Part model, mm, in its own coordinate system. A direction names the side the tool comes from. Give positions to 0.01 mm unless a question says otherwise; leave off trailing zeros. Order: outer loops, then holes, each group sorted by start corner. A loop starts at its lowest first (then second) coordinate and runs counter-clockwise, first axis right, second up.
1. Slice it at D-D on y = 29. List the corners of the cut face in (x, z).
2. Slice it at B-B on y = 0. List the corners of the cut face in (x, z).
3. Slice it at C-C on x = -34.43. List the corners of the cut face in (y, z).
4. Slice it at A-A on x = -0.5. List the corners of the cut face in (y, z), and give its area (3 significant figures).
5. Drop flat-ended pins along their axis: pin 1 Ø5 at (y, z) = (38, 3.5) entering from +X; pin 2 Ø2.5 at (x, z) = (-5, 3) entering from +Y; pin 3 Ø4 at (y, z) = (38.5, 5) entering from -X. Give the stop position or say it passes through.
6. Mould opens along X. For faces 6 (the flat face through (22, 52, 4)), 7 (the flat face through (0, 41, 4)), 8 (the flat face through (7, -7, 2)), 9 (the flat face through (-22, 52, 4)) say: +X half, -X half, draft (parallel to the pull), parting line (faces both ways), or undercut.
7. Which spindle directions (+Z, -Z, +X, -X, +Y, -Y) get a long thin tool onto all of the face, cutting with end or side? Do faces 1 (the cylindrical face through (9.824, 3.094, 1.458)), 2 (the flat face through (-1, 14, 0)), 3 (the cylindrical face through (4.38, -8.43, 0.46)), 4 (the flat face through (-15, 14, 6)), 5 (the flat face through (13, 46, 4)). Say none if no direction does.
8. Probe line 1 (Y direction, x = -45.5, z = 7.75); line 2 (Y direction, x = 15, z = 2); line 3 (Y direction, x = 16, z = 3.15). List the from-to ranges inside material, lowest first.
from build123d import *

# Parameters (mm, degrees)
SKETCH_2_W                = 100
SKETCH_2_H                = 40
EXTRUDE_1_DEPTH           = 6
SKETCH_5_W                = 100
SKETCH_5_H                = 40
EXTRUDE_2_DEPTH           = 3
SKETCH_6_R                = 9.5
CUT_EXTRUDE_1_DEPTH       = 7
CUT_EXTRUDE_START         = -8
SKETCH_7_R                = 9.5
CUT_EXTRUDE_2_DEPTH       = 8
SKETCH_8_R                = 10.3
CUT_EXTRUDE_3_DEPTH       = 1.1
SKETCH_9_R                = 1.5
CUT_EXTRUDE_4_DEPTH       = 15
SKETCH_11_W               = 100
SKETCH_11_H               = 9
EXTRUDE_5_DEPTH           = 8
FILLET_3_R                = 5
SKETCH_16_R               = 1.5
CUT_EXTRUDE_6_DEPTH       = 10
HOLE_WIZARD_5_D           = 3
HOLE_WIZARD_5_CBORE_D     = 5.5
HOLE_WIZARD_5_CBORE_DEPTH = 3
SKETCH_20_R               = 1.5
CUT_EXTRUDE_7_DEPTH       = 10
SKETCH_22_R               = 9.5
SKETCH_22_R_2             = 8.5
EXTRUDE_6_DEPTH           = 2
SKETCH_23_W               = 46
SKETCH_23_H               = 8
EXTRUDE_7_DEPTH           = 25
SKETCH_24_W               = 13
SKETCH_24_H               = 8
CUT_EXTRUDE_8_DEPTH       = 12
CHAMFER_1_SIZE            = 2
FILLET_4_R                = 4
SKETCH_25_R               = 1.5
CUT_EXTRUDE_9_DEPTH       = 91.65870063


with BuildPart() as part:
    # 草图2 → 凸台-拉伸1 (new body)
    with BuildSketch(Plane.XY):
        Rectangle(SKETCH_2_W, SKETCH_2_H)
    extrude(amount=EXTRUDE_1_DEPTH)

    # 草图5 → 凸台-拉伸2 (add)
    with BuildSketch(Plane.XY.offset(6)):
        Rectangle(SKETCH_5_W, SKETCH_5_H)
    extrude(amount=EXTRUDE_2_DEPTH)

    # 草图6 → 切除-拉伸1 (cut)
    with BuildSketch(Plane.XY.offset(9)):
        Circle(SKETCH_6_R)
    extrude(amount=-CUT_EXTRUDE_1_DEPTH, mode=Mode.SUBTRACT)

    # 草图7 → 切除-拉伸2 (cut)
    with BuildSketch(Plane(origin=(0, 0, 0), x_dir=(-1, 0, 0), z_dir=(0, 0, -1)).offset(CUT_EXTRUDE_START)):
        with Locations(Location((0, 0, 0), (0, 0, 180))):
            Circle(SKETCH_7_R)
    extrude(amount=CUT_EXTRUDE_2_DEPTH, mode=Mode.SUBTRACT)

    # 草图8 → 切除-拉伸3 (cut)
    with BuildSketch(Plane.XY.offset(2)):
        Circle(SKETCH_8_R)
    extrude(amount=-CUT_EXTRUDE_3_DEPTH, mode=Mode.SUBTRACT)

    # 草图9 → 切除-拉伸4 (cut)
    with BuildSketch(Plane(origin=(0, 0, 0), x_dir=(-1, 0, 0), z_dir=(0, 0, -1))):
        with Locations((-15.07, 5)):
            Circle(SKETCH_9_R)
        with Locations((34.43, 5)):
            Circle(SKETCH_9_R)
        with Locations((-15.07, -5)):
            Circle(SKETCH_9_R)
        with Locations((34.43, -5)):
            Circle(SKETCH_9_R)
    extrude(amount=-CUT_EXTRUDE_4_DEPTH, mode=Mode.SUBTRACT)

    # 草图11 → 凸台-拉伸5 (add)
    with BuildSketch(Plane(origin=(0, 20, 0), x_dir=(1, 0, 0), z_dir=(0, 1, 0))):
        with Locations((0, -4.5)):
            Rectangle(SKETCH_11_W, SKETCH_11_H)
    extrude(amount=EXTRUDE_5_DEPTH)

    # 圆角3
    fillet_3_edges = [part.edges().sort_by_distance(p)[0] for p in [
        (-50, 28, 4.5),
        (50, 28, 4.5),
        (50, -20, 4.5),
        (-50, -20, 4.5),
    ]]
    fillet(fillet_3_edges, radius=FILLET_3_R)

    # 草图16 → 切除-拉伸6 (cut)
    with BuildSketch(Plane(origin=(0, 0, 0), x_dir=(-1, 0, 0), z_dir=(0, 0, -1))):
        with Locations((-6, 15.6)):
            Circle(SKETCH_16_R)
        with Locations((6, 15.6)):
            Circle(SKETCH_16_R)
        with Locations((-16, 15.6)):
            Circle(SKETCH_16_R)
        with Locations((16, 15.6)):
            Circle(SKETCH_16_R)
    extrude(amount=-CUT_EXTRUDE_6_DEPTH, mode=Mode.SUBTRACT)

    # 孔5 (through all)
    with Locations(Plane(origin=(-16, 15.6, 9), x_dir=(1, 0, 0), z_dir=(0, 0, 1))):
        with Locations((0, 0), (10, 0), (22, 0), (32, 0)):
            CounterBoreHole(HOLE_WIZARD_5_D / 2, HOLE_WIZARD_5_CBORE_D / 2, HOLE_WIZARD_5_CBORE_DEPTH)

    # 草图20 → 切除-拉伸7 (cut)
    with BuildSketch(Plane(origin=(0, 0, 0), x_dir=(-1, 0, 0), z_dir=(0, 0, -1))):
        with Locations((-46, 24)):
            Circle(SKETCH_20_R)
        with Locations((46, 24)):
            Circle(SKETCH_20_R)
        with Locations((-46, -16)):
            Circle(SKETCH_20_R)
        with Locations((46, -16)):
            Circle(SKETCH_20_R)
    extrude(amount=-CUT_EXTRUDE_7_DEPTH, mode=Mode.SUBTRACT)

    # 草图22 → 凸台-拉伸6 (add)
    with BuildSketch(Plane.XY.offset(9)):
        Circle(SKETCH_22_R)
        Circle(SKETCH_22_R_2, mode=Mode.SUBTRACT)
    extrude(amount=-EXTRUDE_6_DEPTH)

    # 草图23 → 凸台-拉伸7 (add)
    with BuildSketch(Plane(origin=(0, 28, 0), x_dir=(1, 0, 0), z_dir=(0, 1, 0))):
        with Locations((0, -4)):
            Rectangle(SKETCH_23_W, SKETCH_23_H)
    extrude(amount=EXTRUDE_7_DEPTH)

    # 草图24 → 切除-拉伸8 (cut)
    with BuildSketch(Plane(origin=(0, 53, 0), x_dir=(1, 0, 0), z_dir=(0, 1, 0))):
        with Locations((-6.5, -4)):
            Rectangle(SKETCH_24_W, SKETCH_24_H)
        with Locations((6.5, -4)):
            Rectangle(SKETCH_24_W, SKETCH_24_H)
    extrude(amount=-CUT_EXTRUDE_8_DEPTH, mode=Mode.SUBTRACT)

    # 倒角1
    chamfer_1_edges = [part.edges().sort_by_distance(p)[0] for p in [
        (-23, 53, 4),
        (23, 53, 4),
    ]]
    chamfer(chamfer_1_edges, length=CHAMFER_1_SIZE)

    # 圆角4
    fillet_4_edges = [part.edges().sort_by_distance(p)[0] for p in [
        (17, 53, 8),
        (17, 53, 0),
        (-17, 53, 8),
        (-17, 53, 0),
    ]]
    fillet(fillet_4_edges, radius=FILLET_4_R - 0.0001)  # a hair under: the kernel refuses the full size

    # 草图25 → 切除-拉伸9 (cut, through all)
    with BuildSketch(Plane(origin=(23, 0, 0), x_dir=(0, 0, -1), z_dir=(1, 0, 0))):
        with Locations((-4, 48)):
            Circle(SKETCH_25_R)
    extrude(amount=-CUT_EXTRUDE_9_DEPTH, mode=Mode.SUBTRACT)


solid = part.part
Data:
1. outline: (-23, 0) - (23, 0) - (23, 8) - (-23, 8) - close
2. outline: (-50, 0) - (-9.5, 0) - (-9.5, 0.9) - (-10.3, 0.9) - (-10.3, 2) - (-9.5, 2) - (-9.5, 7) - (-8.5, 7) - (-8.5, 9) - (-50, 9) - close; (8.5, 7) - (9.5, 7) - (9.5, 2) - (10.3, 2) - (10.3, 0.9) - (9.5, 0.9) - (9.5, 0) - (50, 0) - (50, 9) - (8.5, 9) - close
3. outline: (-20, 0) - (-6.5, 0) - (-6.5, 9) - (-20, 9) - close; (-3.5, 0) - (3.5, 0) - (3.5, 9) - (-3.5, 9) - close; (6.5, 0) - (28, 0) - (28, 9) - (6.5, 9) - close
4. outline: (-20, 0) - (-9.49, 0) - (-9.49, 0.9) - (-10.29, 0.9) - (-10.29, 2) - (-9.49, 2) - (-9.49, 7) - (-8.49, 7) - (-8.49, 9) - (-20, 9) - close; (8.49, 7) - (9.49, 7) - (9.49, 2) - (10.29, 2) - (10.29, 0.9) - (9.49, 0.9) - (9.49, 0) - (41, 0) - (41, 8) - (28, 8) - (28, 9) - (8.49, 9) - close
4. area: 367 mm2
5. pin 1: stops at x = 23
5. pin 2: stops at y = 41
5. pin 3: stops at x = -23
6. face 6: +X half
6. face 7: undercut
6. face 8: undercut
6. face 9: -X half
7. face 1: none
7. face 2: -Z, +X, -X, +Y, -Y
7. face 3: -Z
7. face 4: +Z
7. face 5: +Z, -Z, +Y
8. line 1: y = -19.97 to -17.41, -14.59 to 22.59, 25.41 to 27.97
8. line 2: y = -20 to -6.5, -3.5 to 3.5, 6.5 to 14.48, 16.72 to 52.46
8. line 3: y = -20 to -6.18, -3.82 to 3.82, 6.18 to 14.1, 17.1 to 46.76, 49.24 to 52.91
